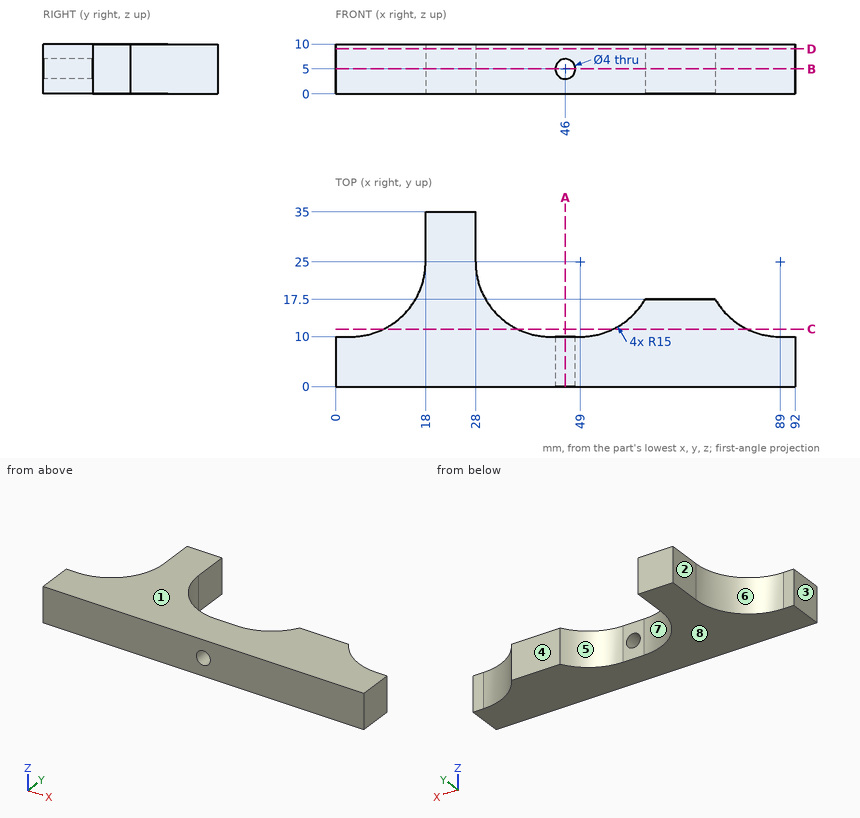
Geometry check sheet. Reference: drawing and pictorial views, mm from the part's lowest x, y, z. A direction names the side the tool comes from. Coordinates: 2 decimals unless noted, no trailing zeros. Loops run counter-clockwise (first coordinate to the right, second up) from the corner with the lowest first, then second, coordinate; pieces in that order, holes last. Notation, with made-up numbers: (44, 80.5) - (86, 80.5) arc R29 ccw to (86, 112.5) - close; hole circle Ø4 at (-6.75, -11). An arc over 180 degrees is marked (long way). Return JSON: item names as keys, results as strings.
1. Tool access check on the marked faces 1, 2, 3, 4 and 5. Record the directions out of +Z, -Z, +X, -X, +Y, -Y that give a thin tool (end or side, any length) a straight path to the whole face; none if there is none.
Established:
{"face 1": "+Z, +X, -X, +Y, -Y", "face 2": "+Z, -Z, -X, +Y", "face 3": "+Z, -Z, -X, +Y, -Y", "face 4": "+Z, -Z, +X, +Y", "face 5": "+Z, -Z, +Y"}
2. Go/stop test with flat-tipped pins: pin 1 (1.5 mm diameter, centred on y = 16, z = 8, fed in from -X); pin 2 (1.5 mm diameter, centred on x = 90.5, z = 4.5, fed in from +Y); pin 3 (2 mm diameter, centred on y = 16, z = 1, fed in from +X); pin 4 (1 mm diameter, centred on x = 24.5, z = 7, fed in from -Y). Record where each tip stops, or that it passes through.
Established:
{"pin 1": "stops at x = 14.4", "pin 2": "stops at y = 10", "pin 3": "stops at x = 77.82", "pin 4": "stops at y = 0"}
3. Section check B-B, the plane z = 5. Record the boundary of the cut face in (x, y).
Established:
{"outline": "(0, 0) - (44, 0) - (44, 10) - (43, 10) arc R15 cw to (28, 25) - (28, 35) - (18, 35) - (18, 25) arc R15 cw to (3, 10) - (0, 10) - close; (48, 0) - (92, 0) - (92, 10) - (89, 10) arc R15 cw to (76.01, 17.5) - (61.99, 17.5) arc R15 cw to (49, 10) - (48, 10) - close"}
4. Section check A-A, the plane x = 46. Record the boundary of the cut face in (y, z).
Established:
{"outline": "(0, 0) - (10, 0) - (10, 3) - (0, 3) - close; (0, 7) - (10, 7) - (10, 10) - (0, 10) - close"}
5. Section check C-C, the plane y = 11.5. Record the boundary of the cut face in (x, z), then the cut area to 3 significant figures.
Established:
{"outline": "(9.54, 0) - (36.46, 0) - (36.46, 10) - (9.54, 10) - close; (55.54, 0) - (82.46, 0) - (82.46, 10) - (55.54, 10) - close", "area": "538 mm2"}
6. Section check D-D, the plane z = 9. Record the boundary of the cut face in (x, y), then the cut area to 3 significant figures.
Established:
{"outline": "(0, 0) - (92, 0) - (92, 10) - (89, 10) arc R15 cw to (76.01, 17.5) - (61.99, 17.5) arc R15 cw to (49, 10) - (43, 10) arc R15 cw to (28, 25) - (28, 35) - (18, 35) - (18, 25) arc R15 cw to (3, 10) - (0, 10) - close", "area": "1,430 mm2"}
7. Thickness scan on L1, parallel to Z at x = 46, y = 5.5; L2, parallel to X at y = 3, z = 5.25; L3, parallel to Y at x = 71, z = 4. Record the ranges inside material, lowest first.
Established:
{"L1": "z = 0 to 3, 7 to 10", "L2": "x = 0 to 44.02, 47.98 to 92", "L3": "y = 0 to 17.5"}
8. Mould release check, pull along X, two halves, no side actions. Record for the marked faces 6, 7 and 8: +X half, -X half, draft (parallel to the pull), parting line (faces both ways), or undercut.
Established:
{"face 6": "-X half", "face 7": "undercut", "face 8": "draft"}
